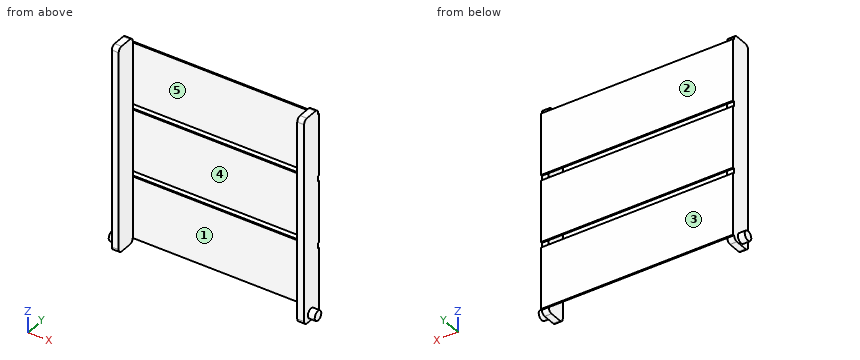
```python
from build123d import *

# Parameters (mm, degrees)
BOSS_EXTRUDE1_DEPTH = 50
SKETCH2_W           = 1400
SKETCH2_H           = 450
BOSS_EXTRUDE2_DEPTH = 10
LPATTERN1_COUNT     = 2
LPATTERN1_PITCH     = 1350
LPATTERN2_COUNT     = 3
LPATTERN2_PITCH     = 490
SKETCH3_R           = 35
BOSS_EXTRUDE3_DEPTH = 50
LPATTERN3_COUNT     = 2
LPATTERN3_PITCH     = 1450


with BuildPart() as part:
    # Sketch1 → Boss-Extrude1 (new body)
    with BuildSketch(Plane(origin=(0, 0, 0), x_dir=(0, 0, -1), z_dir=(1, 0, 0))):
        with BuildLine():
            Line((-720, -75), (720, -75))
            ThreePointArc((720, -75), (741.213203436, -66.213203436), (750, -45))
            Line((750, -45), (750, 45))
            ThreePointArc((750, 45), (741.213203436, 66.213203436), (720, 75))
            Line((720, 75), (-720, 75))
            ThreePointArc((-720, 75), (-741.213203436, 66.213203436), (-750, 45))
            Line((-750, 45), (-750, -45))
            ThreePointArc((-750, -45), (-741.213203436, -66.213203436), (-720, -75))
        make_face()
    boss_extrude1 = extrude(amount=BOSS_EXTRUDE1_DEPTH)

    # Sketch2 → Boss-Extrude2 (add)
    with BuildSketch(Plane(origin=(0, 75, 0), x_dir=(1, 0, 0), z_dir=(0, 1, 0))):
        with Locations((700, 495)):
            Rectangle(SKETCH2_W, SKETCH2_H)
    boss_extrude2 = extrude(amount=BOSS_EXTRUDE2_DEPTH)

    # LPattern1: Boss-Extrude1 ×2
    with Locations(*[(i * LPATTERN1_PITCH, 0, 0) for i in range(1, LPATTERN1_COUNT)]):
        add(boss_extrude1)

    # LPattern2: Boss-Extrude2 ×3
    with Locations(*[(0, 0, i * LPATTERN2_PITCH) for i in range(1, LPATTERN2_COUNT)]):
        add(boss_extrude2)

    # Sketch3 → Boss-Extrude3 (add)
    with BuildSketch(Plane.ZY):
        with Locations(Location((-700, 0, 0), (0, 0, 180))):
            Circle(SKETCH3_R)
    boss_extrude3 = extrude(amount=BOSS_EXTRUDE3_DEPTH)

    # LPattern3: Boss-Extrude3 ×2
    with Locations(*[(i * LPATTERN3_PITCH, 0, 0) for i in range(1, LPATTERN3_COUNT)]):
        add(boss_extrude3)


solid = part.part
```
Can you work these out from the model? Positions are in its coordinate system, mm. Face numbers are marked on the shaded views. A direction names the side the tool comes from. Round coordinates to 2 decimals unless told otherwise and drop trailing zeros. Loops run counter-clockwise (first coordinate to the right, second up) from the corner with the lowest first, then second, coordinate; pieces in that order, holes last. Notation, with made-up numbers: (-14, 53) -> (45, 53) arc R25 ccw to (45, 71) -> close; hole circle Ø6 at (74, 62.25). An arc over 180 degrees is marked (long way). Answer in a Markdown table with one row per item.
Item 1: Suppose I cut it at B-B, the plane y = 0. List the corners of the cut face in (x, z) for me, plus the area to 3 significant figures.
Answer block:
| item | result |
|---|---|
| outline | (-50, -735) -> (0, -735) -> (0, -750) -> (50, -750) -> (50, 750) -> (0, 750) -> (0, -665) -> (-50, -665) -> close; (1350, -750) -> (1400, -750) -> (1400, -735) -> (1450, -735) -> (1450, -665) -> (1400, -665) -> (1400, 750) -> (1350, 750) -> close |
| area | 157,000 mm² |
Item 2: Suppose I cut it at D-D, the plane z = -700. List the corners of the cut face in (x, y) for me.
Answer block:
| item | result |
|---|---|
| outline | (-50, -35) -> (0, -35) -> (0, -75) -> (50, -75) -> (50, 75) -> (1350, 75) -> (1350, -75) -> (1400, -75) -> (1400, -35) -> (1450, -35) -> (1450, 35) -> (1400, 35) -> (1400, 85) -> (0, 85) -> (0, 35) -> (-50, 35) -> close |
Item 3: Suppose I cut it at C-C, the plane z = 79. List the corners of the cut face in (x, y) for me, plus the area to 3 significant figures.
Answer block:
| item | result |
|---|---|
| outline | (0, -75) -> (50, -75) -> (50, 75) -> (1350, 75) -> (1350, -75) -> (1400, -75) -> (1400, 85) -> (0, 85) -> close |
| area | 29,000 mm² |
Item 4: On a 3-axis mill with a long thin cutter (end or side, diameter ignored), from which of +Z, -Z, +X, -X, +Y, -Y can I reach the whole of each face in a straight line? I mean the marked faces 1 and 2. Say none if no direction works.
Answer block:
| item | result |
|---|---|
| face 1 | +Z, -Z, -Y |
| face 2 | +Z, -Z, +X, -X, +Y |
Item 5: We'd pull the mould along X, two halves only. Please class the marked faces 3, 4 and 5: released by +X, released by -X, zero draft, split by the parting line, or undercut.
Answer block:
| item | result |
|---|---|
| face 3 | zero draft |
| face 4 | undercut |
| face 5 | undercut |
Item 6: Will these pins go through, and if not, where does the flat tip stop? P1, Ø3, axis at x = 457, y = 82, coming from the +Z side; P2, Ø2, axis at y = 8.5, z = 33, coming from the +X side; P3, Ø5, axis at x = 751.5, y = 79, coming from the -Z side.
Answer block:
| item | result |
|---|---|
| P1 | z = 710 |
| P2 | x = 1400 |
| P3 | z = -720 |
Item 7: Suppose I cut it at A-A, the plane x = 463. List the corners of the cut face in (y, z) for me, plus the area to 3 significant figures.
Answer block:
| item | result |
|---|---|
| outline | (75, -720) -> (85, -720) -> (85, -270) -> (75, -270) -> close; (75, -230) -> (85, -230) -> (85, 220) -> (75, 220) -> close; (75, 260) -> (85, 260) -> (85, 710) -> (75, 710) -> close |
| area | 13,500 mm² |
Item 8: If I drill on probe 1 along X at (y, z) = (-53, -243); probe 2 along Y at (x, z) = (615.5, -633); probe 3 along Z at (x, y) = (40.5, 65), over which ranges is the centre line in solid material (lowest first)?
Answer block:
| item | result |
|---|---|
| probe 1 | 0 to 50, 1350 to 1400 |
| probe 2 | 75 to 85 |
| probe 3 | -742.36 to 742.36 |
